from build123d import *

# Parameters (mm, degrees)
F0_W     = 400
F0_H     = 350
F1_DEPTH = 19
F3_DEPTH = 19.001
F4_DEPTH = 19.001


with BuildPart() as f1:
    # F0 (on Top) → F1 (new body)
    with BuildSketch(Plane.XY):
        Rectangle(F0_W, F0_H)
    extrude(amount=F1_DEPTH)

    # F2 (on face) → F3 (cut, through all)
    with BuildSketch(Plane.XY.offset(19)):
        Polygon((66.666667, -137.436854), (-200, 0), (-200, -175), (200, -175), (200, -68.718427), align=None)
    extrude(amount=-F3_DEPTH, mode=Mode.SUBTRACT)

    # F2 (on face) → F4 (cut, through all)
    with BuildSketch(Plane.XY.offset(19)):
        Polygon((-200, 175), (-200, 0), (66.666667, 137.436854), (200, 68.718427), (200, 175), align=None)
    extrude(amount=-F4_DEPTH, mode=Mode.SUBTRACT)


solid = f1.part
Build history of the part. All positions in model axes, mm. Round coordinates to 2 decimals unless told otherwise and drop trailing zeros. Write each loop counter-clockwise with the first axis right and the second up, starting at its lowest first coordinate (ties: lowest second). Pieces come first, ordered by that corner, then holes. Notation, with made-up numbers: M 1.5,79 L 37.5,79 A24 ccw 37.5,94 Z; hole C 3,71 d6. An arc over 180 degrees is marked long. Use CSV: the item, a comma, the result in double quotes.
1. Saw through at B-B (y = 117.5). Give the cut face in (x, z).
Reply:
outline,"M 27.98,0 L 105.35,0 L 105.35,19 L 27.98,19 Z"
2. Saw through at C-C (x = 76.5). Give the cut face in (y, z), plus the area to 3 significant figures.
Reply:
outline,"M -132.37,0 L 132.37,0 L 132.37,19 L -132.37,19 Z"
area,"5,030 mm²"
3. Saw through at A-A (z = 12.5). Give the cut face in (x, y).
Reply:
outline,"M -200,0 L 66.67,-137.44 L 200,-68.72 L 200,68.72 L 66.67,137.44 Z"
4. Flat gauge pins, fed straight in: pin 1 (4 mm diameter, centred on x = -14, z = 13, fed in from +Y); pin 2 (8 mm diameter, centred on x = 97.5, z = 9, fed in from +Y); pin 3 (3 mm diameter, centred on x = -131.5, z = 12.5, fed in from +Y). Where does each tip first touch, or does it go through?
Reply:
pin 1,"stops at y = 96.89"
pin 2,"stops at y = 123.61"
pin 3,"stops at y = 36.08"
5. Wall check: probe 1 along Y at (x, z) = (23, 7.5); probe 2 along Y at (x, z) = (-100.5, 10); probe 3 along X at (y, z) = (122.5, 2.75). Give the ranges that are in metal, low to high. Write a range as from..to.
Reply:
probe 1,"y = -114.93..114.93"
probe 2,"y = -51.28..51.28"
probe 3,"x = 37.68..95.65"
